Input: dimensioned drawing with shaded views. Units: mm. Origin: part minimum x, y, z. A direction names the side the tool comes from. Give positions to 0.01 mm unless a question says otherwise; leave off trailing zeros. Write each loop counter-clockwise with the first axis right and the second up, starting at its lowest first coordinate (ties: lowest second). Pieces come first, ordered by that corner, then holes. Notation, with made-up numbers: (-4.75, 66.25) - (3.25, 66.25) arc R23 cw to (3.25, 95.25) - close; hole circle Ø4 at (57, -30). An arc over 180 degrees is marked (long way). Answer as CSV lines item,"result".
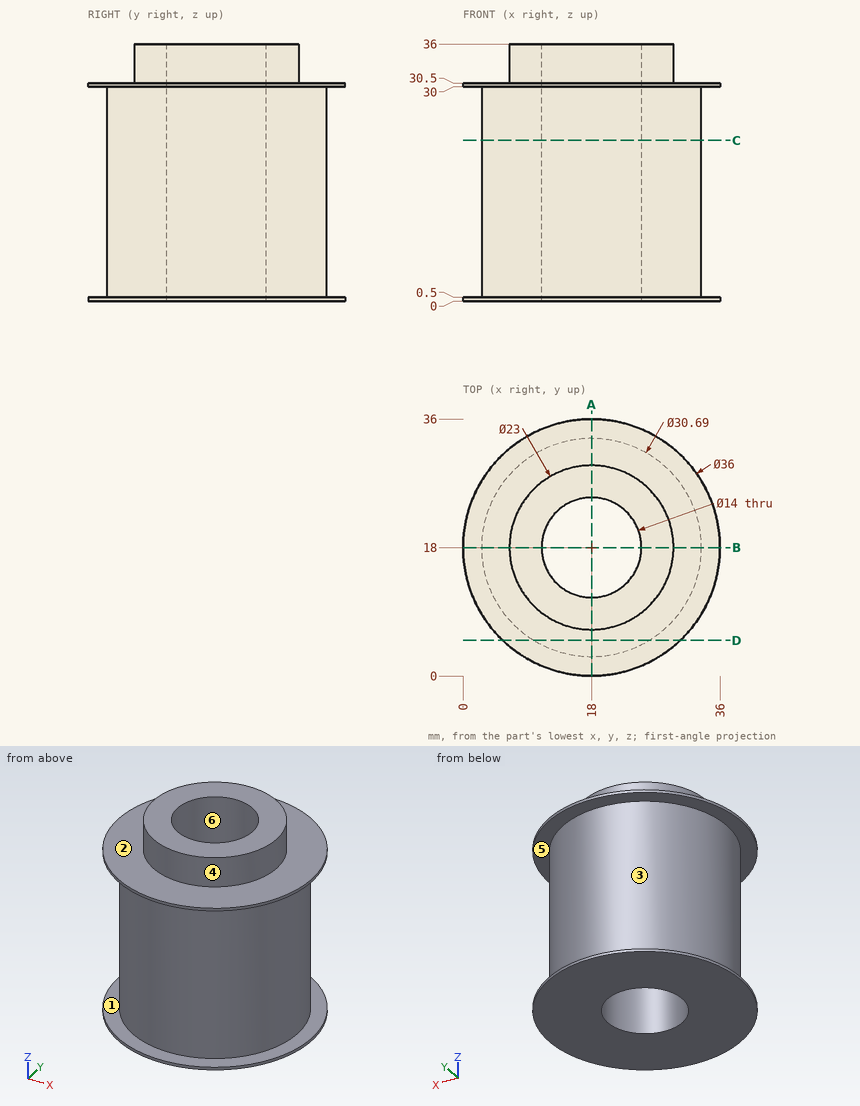
Item 1: Cut plane C-C on z = 22.5. Return the cut outline in (x, y) (3 decimals).
The answers:
outline,"circle Ø30.69 at (18, 18); hole circle Ø14 at (18, 18)"
Item 2: Cut plane A-A on x = 18. Return the cut outline in (y, z) (3 decimals), plus the area to 3 significant figures.
The answers:
outline,"(0, 0) - (11, 0) - (11, 36) - (6.5, 36) - (6.5, 30.5) - (0, 30.5) - (0, 30) - (2.655, 30) - (2.655, 0.5) - (0, 0.5) - close; (25, 0) - (36, 0) - (36, 0.5) - (33.345, 0.5) - (33.345, 30) - (36, 30) - (36, 30.5) - (29.5, 30.5) - (29.5, 36) - (25, 36) - close"
area,"564 mm²"
Item 3: Cut plane D-D on y = 5. Return the cut outline in (x, z), plus the area to 3 significant figures.
The answers:
outline,"(5.55, 0) - (30.45, 0) - (30.45, 0.5) - (26.15, 0.5) - (26.15, 30) - (30.45, 30) - (30.45, 30.5) - (5.55, 30.5) - (5.55, 30) - (9.85, 30) - (9.85, 0.5) - (5.55, 0.5) - close"
area,"506 mm²"
Item 4: Reachability of the marked faces 5 and 6 from +Z, -Z, +X, -X, +Y, -Y: full face, straight path, thin tool, end or side. Return the list, or none.
The answers:
face 5,"none"
face 6,"+Z, -Z"
Item 5: Mould query, pull axis Z, two halves, no side actions, for the marked faces 1, 2, 3 and 4. Classes: +Z half, -Z half, draft (parallel to the pull), parting line (faces both ways), or undercut.
The answers:
face 1,"undercut"
face 2,"+Z half"
face 3,"undercut"
face 4,"draft"
Item 6: Ray query, line 1 (Y direction, x = 18, z = 25) (3 decimals); line 2 (Z direction, x = 4.5, y = 7.5); line 3 (Z direction, x = 16.5, y = 4.5). Return the intervals inside material, ascending. Write a range as from..to.
The answers:
line 1,"2.655..11, 25..33.345"
line 2,"0..0.5, 30..30.5"
line 3,"0..30.5"
Item 7: Contact query for flat-ended pins moving along their axis: pin 1 (6 mm diameter, centred on x = 29, z = 7.5, fed in from -Y); pin 2 (12 mm diameter, centred on y = 19.5, z = 12.5, fed in from -X) (3 decimals); pin 3 (1 mm diameter, centred on x = 13.5, y = 30.5, fed in from +Z); pin 4 (11 mm diameter, centred on x = 18, y = 18, fed in from -Z). Output: stop coordinate, or through.
The answers:
pin 1,"y = 4.91"
pin 2,"x = 2.655"
pin 3,"z = 30.5"
pin 4,"through"
